```python
from build123d import *

# Parameters (mm, degrees)
F0_R         = 12.625
F0_R_2       = 10.375
F0_R_3       = 5
F1_DEPTH     = 15
F2_DEPTH     = 15
F3_R         = 12.6739646699
F4_DEPTH     = 6.6
F6_DEPTH     = 7
F7_T4_DEPTH  = 36.6039255786
F7_S5_R      = 12.6739646699
F7_T6_DEPTH  = 20
F7_T10_DEPTH = 24.210816556
F7_S11_R     = 12.6739646699
F7_T12_DEPTH = 14
F8_T1_DEPTH  = 32.8699146781
F9_T1_DEPTH  = 33.2150521969
F10_SCALE    = 0.79


# Not quite as in the source:
# - a fillet or chamfer that OpenCascade refuses, or shapes differently, is made with other operations: its cross-section is extruded or revolved along the edge and cut away or added
# - a feature names something its author has since deleted; it is built from what else it names


with BuildPart() as f1:
    # F0 (on Top) → F1 (new body)
    with BuildSketch(Plane.XY):
        Circle(F0_R)
        Circle(F0_R_2, mode=Mode.SUBTRACT)
        Circle(F0_R_2)
        Circle(F0_R_3, mode=Mode.SUBTRACT)
    extrude(amount=F1_DEPTH)

    # F0 (on Top) → F2 (join)
    with BuildSketch(Plane.XY):
        Circle(F0_R_3)
        with BuildLine():
            ThreePointArc((2.304625, 2.1105280404), (2.9126944678, 1.1321819366), (3.125, 0))
            ThreePointArc((3.125, 0), (-1.1321819366, -2.9126944678), (-2.304625, 2.1105280404))
            ThreePointArc((-2.304625, 2.1105280404), (0, 3.125), (2.304625, 2.1105280404))
        make_face(mode=Mode.SUBTRACT)
        with BuildLine():
            Line((-2.304625, 2.1105280404), (2.304625, 2.1105280404))
            ThreePointArc((2.304625, 2.1105280404), (0, 3.125), (-2.304625, 2.1105280404))
        make_face()
    extrude(amount=F2_DEPTH)

    # F3 (on face) → F4 (join)
    with BuildSketch(Plane.XY.offset(15)):
        Circle(F3_R)
    extrude(amount=-F4_DEPTH)

    # F5 (on face) → F6 (join)
    with BuildSketch(Plane.XY.offset(15)):
        with BuildLine():
            Line((3.5765423992, 12.0519627893), (-3.921679918, 12.0519627893))
            Line((-3.921679918, 12.0519627893), (-3.921679918, -12.0519627893))
            ThreePointArc((-3.921679918, -12.0519627893), (-3.7494920856, -12.1066382433), (-3.5765423992, -12.1588537667))
            Line((-3.5765423992, -12.1588537667), (3.5765423992, -12.1588537667))
            Line((3.5765423992, -12.1588537667), (3.5765423992, 12.0519627893))
        make_face()
    extrude(amount=F6_DEPTH)

    # F7: fillet of radius 5 on 2 edges, made by hand


with BuildPart() as f7_tool2:
    # F7_s3 → F7_t4 (new body)
    with BuildSketch(Plane.XZ.offset(-12.0519627893)):
        with BuildLine():
            ThreePointArc((-8.921679918, 15), (-5.3861460121, 16.4644660941), (-3.921679918, 20))
            Line((-3.921679918, 20), (-3.921679918, 15))
            Line((-3.921679918, 15), (-8.921679918, 15))
        make_face()
    extrude(amount=F7_T4_DEPTH)

    # F7_s5 → F7_t6 (intersect, symmetric)
    with BuildSketch(Plane.XY.offset(17.5)):
        Circle(F7_S5_R)
    extrude(amount=F7_T6_DEPTH, both=True, mode=Mode.INTERSECT)


with BuildPart() as f1_1:
    add(f1.part)

    # F7_t1: union F7_tool2
    add(f7_tool2.part)


with BuildPart() as f7_tool8:
    # F7_s9 → F7_t10 (new body)
    with BuildSketch(Plane.XZ.offset(12.1588537667)):
        with BuildLine():
            ThreePointArc((8.5765423992, 15), (5.0410084933, 16.4644660941), (3.5765423992, 20))
            Line((3.5765423992, 20), (3.5765423992, 15))
            Line((3.5765423992, 15), (8.5765423992, 15))
        make_face()
    extrude(amount=-F7_T10_DEPTH)

    # F7_s11 → F7_t12 (intersect, symmetric)
    with BuildSketch(Plane.XY.offset(17.5)):
        Circle(F7_S11_R)
    extrude(amount=F7_T12_DEPTH, both=True, mode=Mode.INTERSECT)


with BuildPart() as f1_2:
    add(f1_1.part)

    # F7_t7: union F7_tool8
    add(f7_tool8.part)

    # F8: chamfer of 5 on 1 edges, made by hand

    # F8_s2 → F8_t1 (cut)
    with BuildSketch(Plane.YZ.offset(-16.434957339)):
        Polygon((-12.1588537667, 17), (-7.1588537667, 22), (-12.1588537667, 22), align=None)
    extrude(amount=F8_T1_DEPTH, mode=Mode.SUBTRACT)

    # F9: chamfer of 5 on 1 edges, made by hand

    # F9_s2 → F9_t1 (cut)
    with BuildSketch(Plane.YZ.offset(-16.7800948578)):
        Polygon((12.0519627893, 17), (7.0519627893, 22), (12.0519627893, 22), align=None)
    extrude(amount=F9_T1_DEPTH, mode=Mode.SUBTRACT)


with BuildPart() as f1_3:
    # F10: moved
    add(f1_2.part.scale(F10_SCALE))


solid = f1_3.part
```
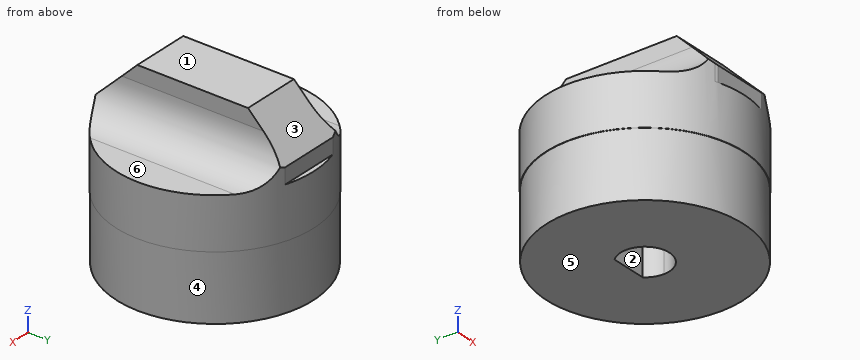
The model under review builds one solid part; all positions refer to its coordinate system, in mm. Face numbers are marked on the shaded views. A direction names the side the tool comes from. Round coordinates to 2 decimals unless told otherwise and drop trailing zeros. Loops run counter-clockwise (first coordinate to the right, second up) from the corner with the lowest first, then second, coordinate; pieces in that order, holes last.
1) Consider section D-D on z = 11.25. State the section outline as (x, y) points.
Values follow:
outline: circle Ø20.02 at (0, 0)
2) Consider section C-C on z = 4.5. State the section outline as (x, y) points.
Values follow:
outline: circle Ø19.95 at (0, 0); hole (-1.82, 1.67) arc R2.47 ccw (long way) to (1.82, 1.67) - close
3) Wall thickness on line 1 along Y through (x, z) = (0, 5.5); line 2 along X through (y, z) = (0, 2.75); line 3 along Z through (x, y) = (-8.5, 2.5): over which ranges is each line inside the solid? List them lowest first.
Values follow:
line 1: y = -9.97 to -2.47, 1.67 to 9.97
line 2: x = -9.97 to -2.47, 2.47 to 9.97
line 3: z = 0 to 11.85
4) Tool access review of the marked faces 5 and 6: name each direction out of +Z, -Z, +X, -X, +Y, -Y from which nothing blocks a thin tool from reaching the whole face with its end or side.
Values follow:
face 5: -Z, +X, -X, +Y, -Y
face 6: +Z, +X, +Y, -Y
5) Clearance check with flat-ended pins moving along their axes: P1, Ø0.8, axis at x = -1, z = 13, coming from the +Y side; P2, Ø1.3, axis at x = 0.5, z = 13, coming from the -Y side; P3, Ø3, axis at y = 2.5, z = 12.5, coming from the -X side. State where each tip first meets the part, or that it passes through.
Values follow:
P1: stops at y = 9.52
P2: stops at y = -9.61
P3: stops at x = -9.95
6) The part is to be moulded in two halves that separate along Y. For the marked faces 1, 2, 3 and 4, say which applies: pulls with the +Y half, pulls with the -Y half, needs draft (parallel to the pull), parting line crosses it, or undercut.
Values follow:
face 1: needs draft
face 2: undercut
face 3: pulls with the +Y half
face 4: parting line crosses it
